The drawing under review shows one solid part. Ordinate dimensions are in mm from its lowest x, y, z. A direction names the side the tool comes from. Give positions to 0.01 mm unless a question says otherwise; leave off trailing zeros. Write each loop counter-clockwise with the first axis right and the second up, starting at its lowest first coordinate (ties: lowest second). Pieces come first, ordered by that corner, then holes.
Q1. We need section A-A (x = 10.5). Write out the cut boundary in (y, z), then the cut area to 3 significant figures.
Q2. Mouldability with a two-part tool opening along Y and no side actions: class the marked faces 3, 4, 5 and 6 as released by +Y, released by -Y, zero draft, split by the parting line, or undercut.
Q3. Insertion check: P1, Ø1.5, axis at x = 17, y = 7, coming from the -Z side. The pin has a flat end and moves straight along its axis. Give the tip position at first contact, or say it passes through.
Q4. We need section C-C (z = 31.5). Write out the cut boundary in (x, y).
Q5. Machinability: for the marked faces 1 and 2, which of the approach directions +Z, -Z, +X, -X, +Y, -Y give a long, thin tool a straight path to every point of the face, cutting with its end or side? Answer none if there is none.
Q6. For line 1 (Y direction, x = 17, z = 21); line 2 (X direction, y = 2.25, z = 30), list the stretches that pass through material, from the lowest coordinate up.
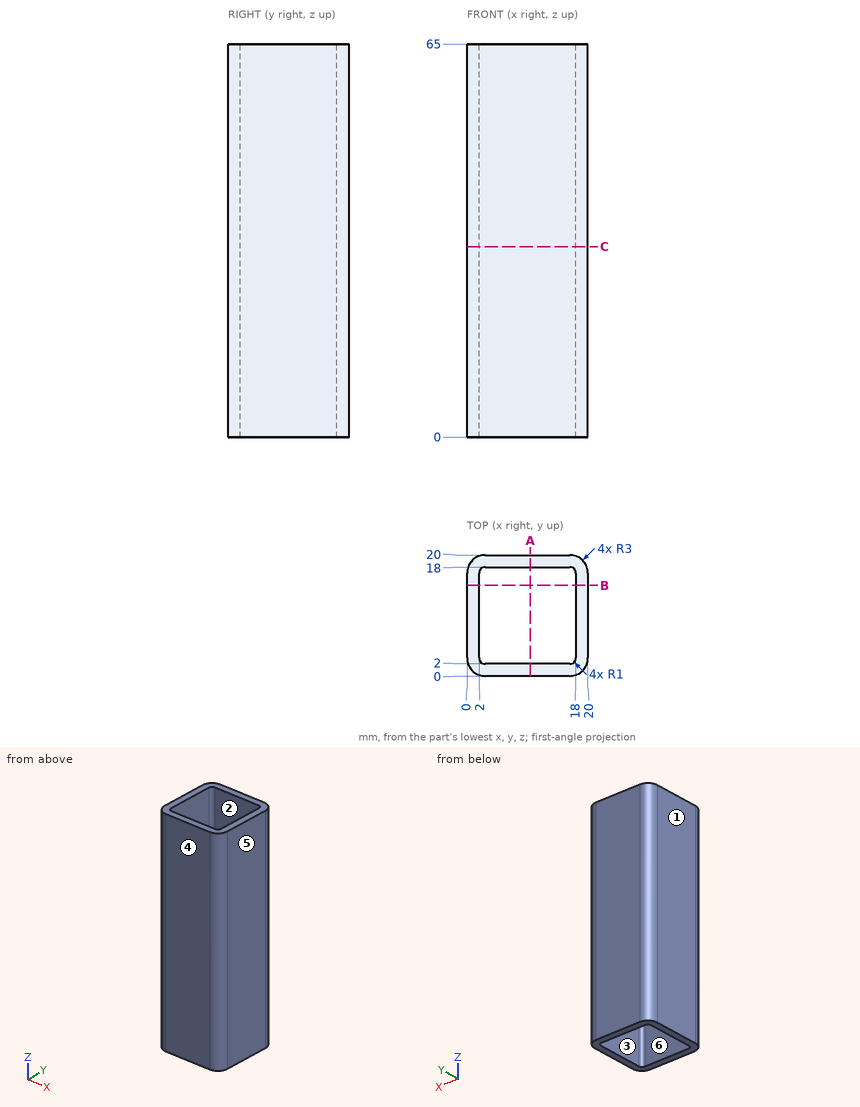
Computed:
1. outline: (0, 0) - (2, 0) - (2, 65) - (0, 65) - close; (18, 0) - (20, 0) - (20, 65) - (18, 65) - close
1. area: 260 mm2
2. face 3: undercut
2. face 4: released by -Y
2. face 5: zero draft
2. face 6: undercut
3. P1: passes through
4. outline: (0, 3) arc R3 ccw to (3, 0) - (17, 0) arc R3 ccw to (20, 3) - (20, 17) arc R3 ccw to (17, 20) - (3, 20) arc R3 ccw to (0, 17) - close; hole (2, 3) arc R1 ccw to (3, 2) - (17, 2) arc R1 ccw to (18, 3) - (18, 17) arc R1 ccw to (17, 18) - (3, 18) arc R1 ccw to (2, 17) - close
5. face 1: +Z, -Z, -X, +Y, -Y
5. face 2: +Z, -Z
6. line 1: y = 0 to 2, 18 to 20
6. line 2: x = 0.1 to 2.34, 17.66 to 19.9
